Geometry check sheet. Reference: drawing and pictorial views, mm from the part's lowest x, y, z. A direction names the side the tool comes from. Round coordinates to 2 decimals unless told otherwise and drop trailing zeros. Loops run counter-clockwise (first coordinate to the right, second up) from the corner with the lowest first, then second, coordinate; pieces in that order, holes last. Notation, with made-up numbers: (30, -21.5) -> (63, -21.5) arc R15 cw to (63, 1.5) -> close; hole circle Ø8 at (82.5, 37). An arc over 180 degrees is marked (long way). Use one line per item in the form item = value. Start each with the question number.
(1) Go/stop test with a flat-tipped pin: pin 1 (5 mm diameter, centred on x = 4, z = 41, fed in from -Y). Record where the tip stops, or that it passes through.
(2) Set-up check for the marked faces 1, 2 and 3: record each of +Z, -Z, +X, -X, +Y, -Y from which the full face is reachable in a straight line by a thin tool's end or side.
(3) Sectioned sample at A-A (y = 16.5). Record the cut outline in (x, z).
(4) Material ranges on probe 1 along Z at (x, y) = (10, 19.5); probe 2 along Y at (x, z) = (4, 27.5); probe 3 along Z at (x, y) = (6.75, 14) (1 decimal), recorded low to high. Write a range as [from, to].
(5) Sectioned sample at C-C (x = 1.5). Record the cut outline in (y, z), and give its area (3 significant figures).
(6) Sectioned sample at D-D (y = 13.5). Record the cut outline in (x, z) (1 decimal).
(7) Draft check along Y on the marked faces 4, 5, 6 and 7. Enter one of: released by +Y, released by -Y, zero draft, split by the parting line, or undercut.
(8) Sectioned sample at B-B (z = 27.5). Record the cut outline in (x, y).
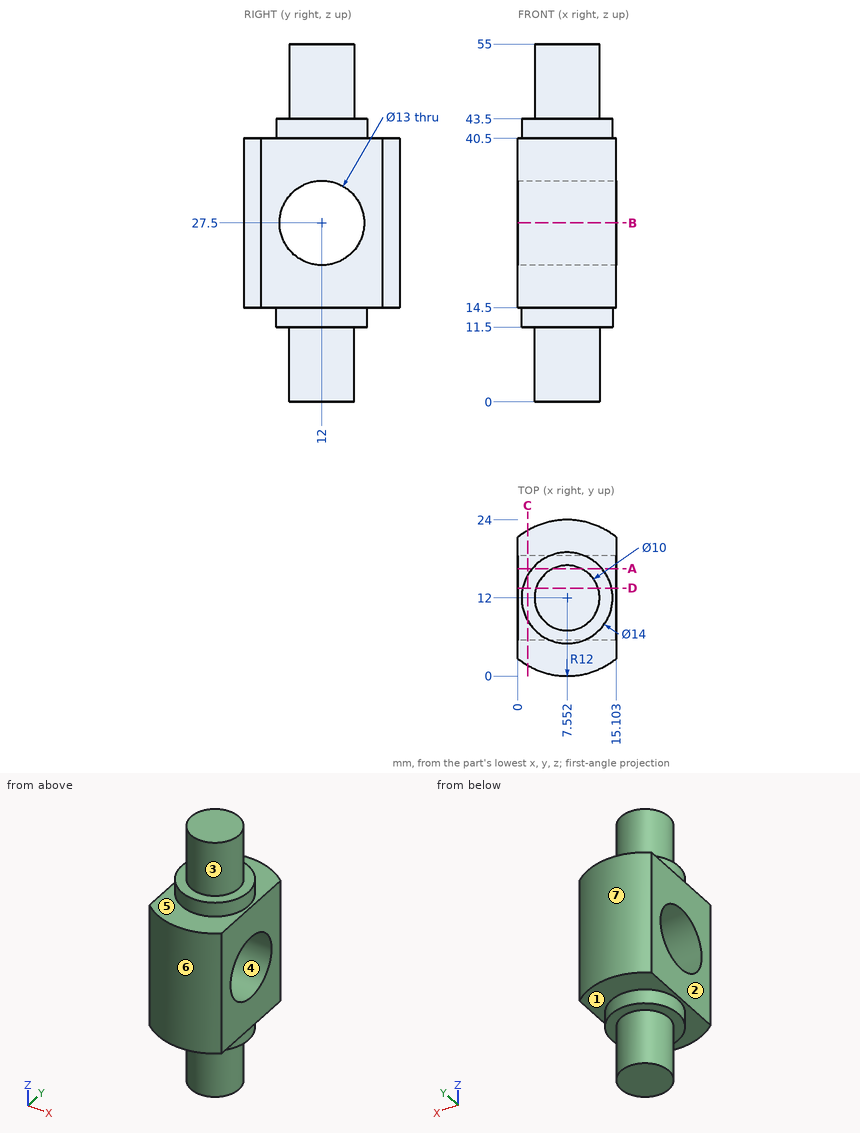
Checks:
q1.pin_1 = 0.05
q2.face_1 = -Z
q2.face_2 = +Z, -Z, -X, +Y, -Y
q2.face_3 = +Z
q3.outline = (0, 14.5) -> (2.19, 14.5) -> (2.19, 11.5) -> (5.37, 11.5) -> (5.37, 0) -> (9.73, 0) -> (9.73, 11.5) -> (12.91, 11.5) -> (12.91, 14.5) -> (15.1, 14.5) -> (15.1, 22.81) -> (0, 22.81) -> close; (0, 32.19) -> (15.1, 32.19) -> (15.1, 40.5) -> (12.91, 40.5) -> (12.91, 43.5) -> (9.73, 43.5) -> (9.73, 55) -> (5.37, 55) -> (5.37, 43.5) -> (2.19, 43.5) -> (2.19, 40.5) -> (0, 40.5) -> close
q4.probe_1 = [14.5, 40.5]
q4.probe_2 = [0.54, 5.5], [18.5, 23.46]
q4.probe_3 = [0, 21.3], [33.7, 55]
q5.outline = (1.64, 14.5) -> (8.48, 14.5) -> (8.48, 11.5) -> (15.52, 11.5) -> (15.52, 14.5) -> (22.36, 14.5) -> (22.36, 40.5) -> (15.52, 40.5) -> (15.52, 43.5) -> (8.48, 43.5) -> (8.48, 40.5) -> (1.64, 40.5) -> close; hole circle Ø13 at (12, 27.5)
q5.area = 448 mm2
q6.outline = (0, 14.5) -> (0.7, 14.5) -> (0.7, 11.5) -> (2.8, 11.5) -> (2.8, 0) -> (12.3, 0) -> (12.3, 11.5) -> (14.4, 11.5) -> (14.4, 14.5) -> (15.1, 14.5) -> (15.1, 21.2) -> (0, 21.2) -> close; (0, 33.8) -> (15.1, 33.8) -> (15.1, 40.5) -> (14.4, 40.5) -> (14.4, 43.5) -> (12.3, 43.5) -> (12.3, 55) -> (2.8, 55) -> (2.8, 43.5) -> (0.7, 43.5) -> (0.7, 40.5) -> (0, 40.5) -> close
q7.face_4 = undercut
q7.face_5 = zero draft
q7.face_6 = released by -Y
q7.face_7 = released by +Y
q8.outline = (0, 2.67) arc R12 ccw to (15.1, 2.67) -> (15.1, 5.5) -> (0, 5.5) -> close; (0, 18.5) -> (15.1, 18.5) -> (15.1, 21.33) arc R12 ccw to (0, 21.33) -> close
